Here's how the part is built. I have some questions about the finished solid (model axes, mm). A direction names the side the tool comes from. Round coordinates to 2 decimals unless told otherwise and drop trailing zeros. Order: outer loops, then holes, each group sorted by start corner. A loop starts at its lowest first (then second) coordinate and runs counter-clockwise, first axis right, second up. Notation, with made-up numbers: (31, 28.25) -> (49, 28.25) arc R26 ccw to (49, 61.25) -> close; hole circle Ø2 at (-7, 84.5). An arc over 180 degrees is marked (long way). One line per item, written item: value.
```python
from build123d import *

# Parameters (mm, degrees)
F2_SIZE  = 0.5
F4_DEPTH = 2.3


with BuildPart() as f1:
    # F0 (on Right) → F1 (revolve)
    with BuildSketch(Plane.YZ):
        Polygon((-2.8, 5), (-2.8, 0), (21.2, 0), (21.2, 2.5), (0, 2.5), (-2.5, 5), align=None)
    revolve(axis=Axis((0, 9.2, 0), (0, 1, 0)))

    # F2
    f2_edges = [f1.edges().sort_by_distance(p)[0] for p in [
        (0, 21.2, -2.5),
    ]]
    chamfer(f2_edges, length=F2_SIZE)

    # F3 (on face) → F4 (cut)
    with BuildSketch(Plane.XZ.offset(2.8)):
        Polygon((0, -1.732051), (1.5, -0.866025), (1.5, 0.866025), (0, 1.732051), (-1.5, 0.866025), (-1.5, -0.866025), align=None)
    extrude(amount=-F4_DEPTH, mode=Mode.SUBTRACT)


solid = f1.part
```
Q1. I want a section at B-B on y = 15.75. Write out the boundary of the cut face in (x, z).
Answers:
outline: circle Ø5 at (0, 0)
Q2. If we mould it in two halves opening along Z, with no side actions, what happens to faces 1 (the face through (-4.88, -2.65, -1.08)), 2 (the face through (-0.76, -1.666, -1.293)), 3 (the face through (-2, -2.8, 0)), 4 (the face through (1.5, -2, 0))? For each: pulls with the +Z half, pulls with the -Z half, needs draft (parallel to the pull), parting line crosses it, or undercut.
Answers:
face 1: parting line crosses it
face 2: undercut
face 3: needs draft
face 4: undercut
Q3. Which directions (+Z, -Z, +X, -X, +Y, -Y) give clear straight access to the entire face, cutting with the end or side of a thin tool? Please do faces 5 (the face through (0, 21.2, 0)), 6 (the face through (0.74, -1.666, -1.305)), 7 (the face through (-2.44, 10.21, -0.54)).
Answers:
face 5: +Z, -Z, +X, -X, +Y
face 6: -Y
face 7: +Y
Q4. I need wall thicknesses on line 1 along X through (y, z) = (8, 0); line 2 along Y through (x, z) = (-0.5, -1); line 3 along Y through (x, z) = (0.5, -3.5). Which ranges of each line are inside material? Lowest first, please.
Answers:
line 1: -2.5 to 2.5
line 2: -0.5 to 21.2
line 3: -2.8 to -1.04
Q5. For P1, Ø2, axis at x = -1, y = 9.5, coming from the -Z side; P2, Ø6, axis at x = 0.5, y = 11.5, coming from the +Z side; P3, Ø0.5, axis at y = -2, z = 0, coming from the -X side; P4, Ø1, axis at x = 3.5, y = 7, coming from the -Z side, each with a flat end and sliding along its axis, tell me the tip position at first contact or that it passes through.
Answers:
P1: z = -2.5
P2: z = 2.5
P3: x = -4.75
P4: through
Q6. I want a section at A-A on z = 0. Write out the boundary of the cut face in (x, y), then the cut area to 3 significant figures.
Answers:
outline: (-5, -2.8) -> (-1.5, -2.8) -> (-1.5, -0.5) -> (1.5, -0.5) -> (1.5, -2.8) -> (5, -2.8) -> (5, -2.5) -> (2.5, 0) -> (2.5, 20.7) -> (2, 21.2) -> (-2, 21.2) -> (-2.5, 20.7) -> (-2.5, 0) -> (-5, -2.5) -> close
area: 121 mm2
